```python
from build123d import *

# Parameters (mm, degrees)
F0_R     = 2.53
F1_DEPTH = 10


with BuildPart() as f1:
    # F0 (on Front) → F1 (new body)
    with BuildSketch(Plane.XZ):
        with BuildLine():
            Line((5, 5), (-5, 5))
            ThreePointArc((-5, 5), (-8.5355339059, 3.5355339059), (-10, 0))
            Line((-10, 0), (-10, -5))
            Line((-10, -5), (10, -5))
            Line((10, -5), (10, 0))
            ThreePointArc((10, 0), (8.5355339059, 3.5355339059), (5, 5))
        make_face()
        with Locations((-5, 0)):
            Circle(F0_R, mode=Mode.SUBTRACT)
        with Locations((5, 0)):
            Circle(F0_R, mode=Mode.SUBTRACT)
    extrude(amount=F1_DEPTH)

    # F3 (on face) → F6 section 0
    with BuildSketch(Plane(origin=(0, 0, 0), x_dir=(-1, 0, 0), z_dir=(0, 1, 0)), mode=Mode.PRIVATE) as f6_s0:
        Polygon((0, -7), (5, -5), (-5, -5), align=None)
    loft([f6_s0.sketch, Vertex(0, -5, -5)])

    # F3 (on face) → F7 section 0
    with BuildSketch(Plane(origin=(0, 0, 0), x_dir=(-1, 0, 0), z_dir=(0, 1, 0)), mode=Mode.PRIVATE) as f7_s0:
        Polygon((5, -5), (10, -7), (10, -5), align=None)
    loft([f7_s0.sketch, Vertex(-10, -5, -5)])

    # F5 (on offset) → F8 section 0
    with BuildSketch(Plane(origin=(0, -5, 0), x_dir=(-1, 0, 0), z_dir=(0, 1, 0)), mode=Mode.PRIVATE) as f8_s0:
        Polygon((5, -7), (10, -5), (0, -5), align=None)
    loft([f8_s0.sketch, Vertex(-5, 0, -5)])

    # F3 (on face) → F9 section 0
    with BuildSketch(Plane(origin=(0, 0, 0), x_dir=(-1, 0, 0), z_dir=(0, 1, 0)), mode=Mode.PRIVATE) as f9_s0:
        Polygon((-10, -7), (-5, -5), (-10, -5), align=None)
    loft([f9_s0.sketch, Vertex(10, -5, -5)])

    # F5 (on offset) → F10 section 0
    with BuildSketch(Plane(origin=(0, -5, 0), x_dir=(-1, 0, 0), z_dir=(0, 1, 0)), mode=Mode.PRIVATE) as f10_s0:
        Polygon((-5, -7), (0, -5), (-10, -5), align=None)
    loft([f10_s0.sketch, Vertex(5, 0, -5)])

    # F2 (on face) → F11 section 0
    with BuildSketch(Plane.XZ.offset(10), mode=Mode.PRIVATE) as f11_s0:
        Polygon((-5, -5), (-10, -5), (-10, -7), align=None)
    loft([f11_s0.sketch, Vertex(-10, -5, -5)])

    # F2 (on face) → F12 section 0
    with BuildSketch(Plane.XZ.offset(10), mode=Mode.PRIVATE) as f12_s0:
        Polygon((10, -5), (5, -5), (10, -7), align=None)
    loft([f12_s0.sketch, Vertex(10, -5, -5)])

    # F2 (on face) → F13 section 0
    with BuildSketch(Plane.XZ.offset(10), mode=Mode.PRIVATE) as f13_s0:
        Polygon((5, -5), (-5, -5), (0, -7), align=None)
    loft([f13_s0.sketch, Vertex(0, -5, -5)])

    # F5 (on offset) → F14 section 0
    with BuildSketch(Plane(origin=(0, -5, 0), x_dir=(-1, 0, 0), z_dir=(0, 1, 0)), mode=Mode.PRIVATE) as f14_s0:
        Polygon((5, -7), (10, -5), (0, -5), align=None)
    loft([f14_s0.sketch, Vertex(-5, -10, -5)])

    # F5 (on offset) → F15 section 0
    with BuildSketch(Plane(origin=(0, -5, 0), x_dir=(-1, 0, 0), z_dir=(0, 1, 0)), mode=Mode.PRIVATE) as f15_s0:
        Polygon((-5, -7), (0, -5), (-10, -5), align=None)
    loft([f15_s0.sketch, Vertex(5, -10, -5)])


solid = f1.part
```
The listing builds one solid part. Answer for the finished solid, in the listing's coordinates (mm). A direction names the side the tool comes from. Coordinates: 2 decimals unless noted, no trailing zeros. Write each loop counter-clockwise with the first axis right and the second up, starting at its lowest first coordinate (ties: lowest second). Pieces come first, ordered by that corner, then holes.
Q1. Section B-B, the plane z = 2.25 is taken. Write down the section's boundary in (x, y), then the cut area to 3 significant figures.
Returned:
outline: (-9.47, -10) - (-6.16, -10) - (-6.16, 0) - (-9.47, 0) - close; (-3.84, -10) - (3.84, -10) - (3.84, 0) - (-3.84, 0) - close; (6.16, -10) - (9.47, -10) - (9.47, 0) - (6.16, 0) - close
area: 143 mm2
Q2. Which of the six approach directions +Z, -Z, +X, -X, +Y, -Y give full straight-line access (tool end or side, diameter ignored) to faces 1 (the cylindrical face through (-8, -5, 4)), 2 (the flat face through (1.78, -1.42, -5.72))?
Returned:
face 1: +Z, -X, +Y, -Y
face 2: -Z
Q3. Given P1, Ø1, axis at x = 6.5, y = -3.5, coming from the +Z side; P2, Ø3, axis at x = -5, z = 0, coming from the -Y side, each flat-ended and moving along its own axis, determine where each tip first touches the part or whether it passes through.
Returned:
P1: stops at z = 4.9
P2: passes through
Q4. Section A-A, the plane y = -7.5 is taken. Write down the section's boundary in (x, z).
Returned:
outline: (-10, -6) - (-7.5, -5) - (-5, -6) - (-2.5, -5) - (0, -6) - (2.5, -5) - (5, -6) - (7.5, -5) - (10, -6) - (10, 0) arc R5 ccw to (5, 5) - (-5, 5) arc R5 ccw to (-10, 0) - close; hole circle Ø5.06 at (-5, 0); hole circle Ø5.06 at (5, 0)
Q5. Section C-C, the plane y = -5.25 is taken. Write down the section's boundary in (x, z).
Returned:
outline: (-10, -5.1) - (-9.75, -5) - (-5, -6.9) - (-0.25, -5) - (0, -5.1) - (0.25, -5) - (5, -6.9) - (9.75, -5) - (10, -5.1) - (10, 0) arc R5 ccw to (5, 5) - (-5, 5) arc R5 ccw to (-10, 0) - close; hole circle Ø5.06 at (-5, 0); hole circle Ø5.06 at (5, 0)
Q6. The mould has two halves that part along X. Classify faces 3 (the flat face through (8.22, -8.58, -5.72)), 4 (the flat face through (1.71, -8.58, -5.75)), 5 (the flat face through (10, -5, -3)), 6 (the flat face through (0, -5, 5)): released by +X, released by -X, zero draft, split by the parting line, or undercut.
Returned:
face 3: undercut
face 4: undercut
face 5: released by +X
face 6: zero draft
Q7. Find the intervals of material crossed by line 1 along X through (y, z) = (-5.25, 2.25); line 2 along Z through (x, y) = (7.25, -8); line 3 along Z through (x, y) = (-5, -6), in increasing order.
Returned:
line 1: x = -9.47 to -6.16, -3.84 to 3.84, 6.16 to 9.47
line 2: z = -5.1 to -1.16, 1.16 to 4.47
line 3: z = -6.6 to -2.53, 2.53 to 5
Q8. Section D-D, the plane x = 1.5 is taken. Write down the section's boundary in (y, z).
Returned:
outline: (-10, -6.4) - (-6.5, -5) - (-5, -5.6) - (-3.5, -5) - (0, -6.4) - (0, 5) - (-10, 5) - close
